Can you work these out from the model? Positions are in its coordinate system, mm. A direction names the side the tool comes from. Coordinates: 2 decimals unless noted, no trailing zeros. Order: outer loops, then holes, each group sorted by start corner. A loop starts at its lowest first (then second) coordinate and runs counter-clockwise, first axis right, second up. Notation, with made-up numbers: (76, -5) -> (93, -5) arc R28 ccw to (93, 28) -> close; hole circle Ø5 at (28, -31). An arc over 180 degrees is marked (long way). Answer in a Markdown table with one row per item. Add a question column.
1. Imagine slicing it at B-B on z = -1.65. Write out the boundary of the cut face in (x, y) (3 decimals).
2. Imagine slicing it at A-A on x = 0. Write out the boundary of the cut face in (y, z) (3 decimals), plus the area to 3 significant figures.
3. If I drill on line 1 along X through (y, z) = (1, -2); line 2 along X through (y, z) = (0.5, 0.7); line 3 along Y through (x, z) = (0, -1.6) (3 decimals), over which ranges is the centre line in solid material (lowest first)? Write a range as [from, to].
4. Imagine slicing it at C-C on y = 0. Write out the boundary of the cut face in (x, z) (3 decimals), plus the area to 3 significant figures.
5. Will these pins go through, and if not, where does the flat tip stop? pin 1 (3 mm diameter, centred on y = -4, z = 0, fed in from +X); pin 2 (1.9 mm diameter, centred on x = -1.5, y = 0.5, fed in from +Z); pin 3 (3.5 mm diameter, centred on x = 0, y = 0, fed in from -Z).
6. On a 3-axis mill with a long thin cutter (end or side, diameter ignored), from which of +Z, -Z, +X, -X, +Y, -Y can I reach the whole of each face in a straight line? I mean faces 4 (the face through (-0.406, 3.095, 1.521)), 5 (the face through (-1, 2, -3)). Say none if no direction works.
7. We'd pull the mould along Y, two halves only. Please class faces 1 (the face through (-44.485, 0.064, -0.042)), 2 (the face through (-45.2, 4.25, -0.04)), 3 (the face through (45.2, -4.25, 0.04)): pulls with the +Y half, pulls with the -Y half, needs draft (parallel to the pull), parting line crosses it, or undercut.
from build123d import *

# Parameters (mm, degrees)
F0_W     = 92
F0_H     = 10.172608
F0_R     = 1.455
F1_DEPTH = 3
F2_R     = 2.794
F3_R     = 3.121392
F4_DEPTH = 3
F5_R     = 1.455
F6_DEPTH = 3


with BuildPart() as f1:
    # F0 (on Top) → F1 (new body, symmetric)
    with BuildSketch(Plane.XY):
        Rectangle(F0_W, F0_H)
        with Locations((-43.031044, 0)):
            Circle(F0_R, mode=Mode.SUBTRACT)
        with Locations((43.108956, 0)):
            Circle(F0_R, mode=Mode.SUBTRACT)
    extrude(amount=F1_DEPTH, both=True)

    # F2
    f2_edges = [f1.edges().sort_by_distance(p)[0] for p in [
        (-46, 5.086304, 0),
        (-46, -5.086304, 0),
        (46, 5.086304, 0),
        (46, -5.086304, 0),
    ]]
    fillet(f2_edges, radius=F2_R)

    # F3 (on face) → F4 (cut, symmetric)
    with BuildSketch(Plane.XY.offset(3)):
        Circle(F3_R)
    extrude(amount=F4_DEPTH, both=True, mode=Mode.SUBTRACT)

    # F5 (on Top) → F6 (cut, symmetric)
    with BuildSketch(Plane.XY):
        Circle(F5_R)
    extrude(amount=F6_DEPTH, both=True, mode=Mode.SUBTRACT)


solid = f1.part
Answers follow:
| question | item | result |
|---|---|---|
| 1 | outline | (-46, -2.292) arc R2.794 ccw to (-43.206, -5.086) -> (43.206, -5.086) arc R2.794 ccw to (46, -2.292) -> (46, 2.292) arc R2.794 ccw to (43.206, 5.086) -> (-43.206, 5.086) arc R2.794 ccw to (-46, 2.292) -> close; hole circle Ø2.91 at (-43.031, 0); hole circle Ø2.91 at (0, 0); hole circle Ø2.91 at (43.109, 0) |
| 2 | outline | (-5.086, -3) -> (-1.455, -3) -> (-1.455, 0) -> (-3.121, 0) -> (-3.121, 3) -> (-5.086, 3) -> close; (1.455, -3) -> (5.086, -3) -> (5.086, 3) -> (3.121, 3) -> (3.121, 0) -> (1.455, 0) -> close |
| 2 | area | 33.6 mm² |
| 3 | line 1 | x = [-46, -44.09], [-41.97, -1.06], [1.06, 42.05], [44.17, 46] |
| 3 | line 2 | x = [-46, -44.4], [-41.66, -3.08], [3.08, 41.74], [44.48, 46] |
| 3 | line 3 | y = [-5.086, -1.455], [1.455, 5.086] |
| 4 | outline | (-46, -3) -> (-44.486, -3) -> (-44.486, 3) -> (-46, 3) -> close; (-41.576, -3) -> (-1.455, -3) -> (-1.455, 0) -> (-3.121, 0) -> (-3.121, 3) -> (-41.576, 3) -> close; (1.455, -3) -> (41.654, -3) -> (41.654, 3) -> (3.121, 3) -> (3.121, 0) -> (1.455, 0) -> close; (44.564, -3) -> (46, -3) -> (46, 3) -> (44.564, 3) -> close |
| 4 | area | 490 mm² |
| 5 | pin 1 | stops at x = 45.99 |
| 5 | pin 2 | stops at z = 0 |
| 5 | pin 3 | stops at z = -3 |
| 6 | face 4 | +Z |
| 6 | face 5 | -Z, +X, -X, +Y, -Y |
| 7 | face 1 | undercut |
| 7 | face 2 | pulls with the +Y half |
| 7 | face 3 | pulls with the -Y half |
